Check sheet for the drawn part. Datum: minimum x, y, z corner. Units: mm. Give positions to 0.01 mm unless a question says otherwise; leave off trailing zeros. Loops run counter-clockwise (first coordinate to the right, second up) from the corner with the lowest first, then second, coordinate; pieces in that order, holes last.
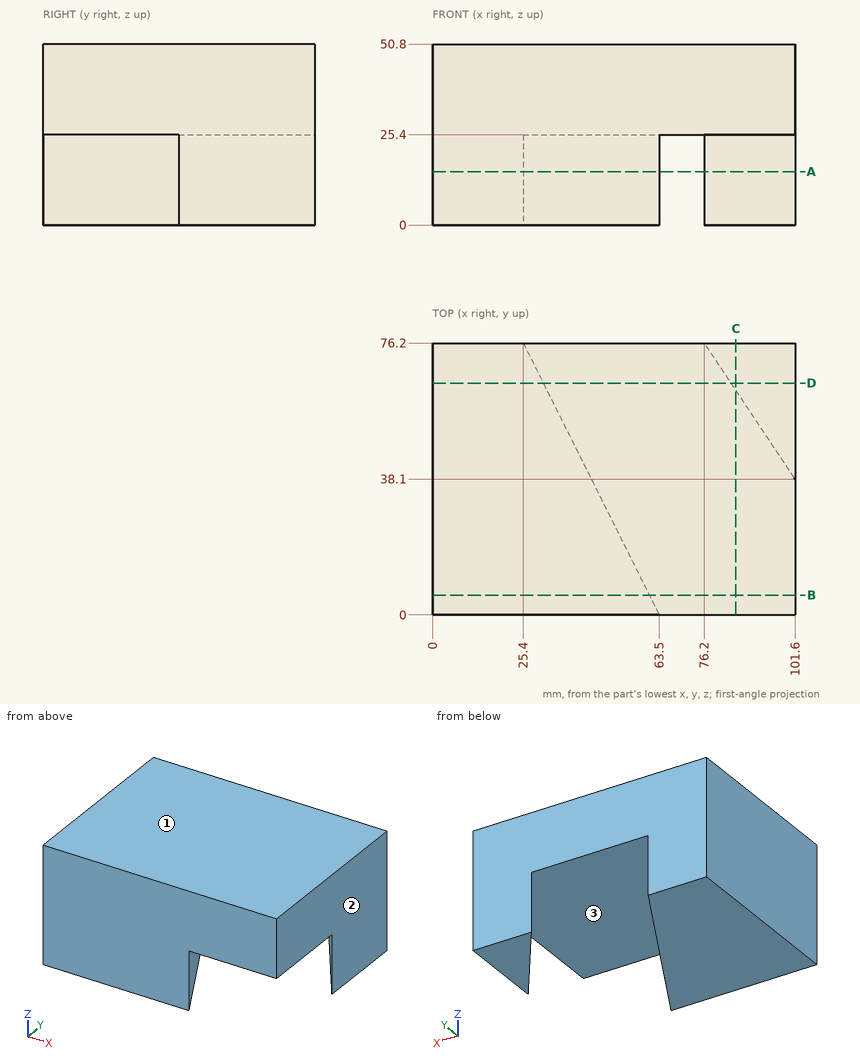
(1) Section check C-C on x = 85. Record the boundary of the cut face in (y, z), plus the area to 3 significant figures.
(2) Section check D-D on y = 65. Record the boundary of the cut face in (x, z).
(3) Section check B-B on y = 5.5. Record the boundary of the cut face in (x, z).
(4) Gauge pin test, flat ends, axial feed: pin 1 Ø2 at (y, z) = (51.5, 23) entering from -X; pin 2 Ø5 at (x, y) = (75.5, 34) entering from -Z; pin 3 Ø4 at (y, z) = (21, 13) entering from +X. Record the tip position at first contact, or that the pin passes through.
(5) Section check A-A on z = 15. Record the boundary of the cut face in (x, y).
(6) Material ranges on line 1 (Z direction, x = 88.5, y = 47.5); line 2 (X direction, y = 67, z = 20); line 3 (Y direction, x = 81.5, z = 24), recorded low to high.
(7) Release check for a two-part mould opening along X. For the marked faces 1, 2 and 3 record: pulls with the +X half, pulls with the -X half, needs draft (parallel to the pull), parting line crosses it, or undercut.
Computed values:
1. outline: (0, 25.4) - (63, 25.4) - (63, 0) - (76.2, 0) - (76.2, 50.8) - (0, 50.8) - close
1. area: 2,270 mm2
2. outline: (0, 0) - (31, 0) - (31, 25.4) - (83.67, 25.4) - (83.67, 0) - (101.6, 0) - (101.6, 50.8) - (0, 50.8) - close
3. outline: (0, 0) - (60.75, 0) - (60.75, 25.4) - (101.6, 25.4) - (101.6, 50.8) - (0, 50.8) - close
4. pin 1: stops at x = 0
4. pin 2: stops at z = 25.4
4. pin 3: stops at x = 54
5. outline: (0, 0) - (63.5, 0) - (25.4, 76.2) - (0, 76.2) - close; (76.2, 76.2) - (101.6, 38.1) - (101.6, 76.2) - close
6. line 1: z = 25.4 to 50.8
6. line 2: x = 0 to 30, 82.33 to 101.6
6. line 3: y = 68.25 to 76.2
7. face 1: needs draft
7. face 2: pulls with the +X half
7. face 3: undercut
